```python
from build123d import *

# Parameters (mm, degrees)
SKETCH2_R               = 76.2
BOSS_EXTRUDE1_DEPTH     = 76.2
SKETCH21_R              = 2.6035
CUT_EXTRUDE4_DEPTH      = 9.525
SKETCH22_R              = 2.6035
CUT_EXTRUDE5_DEPTH      = 9.525
SKETCH27_W              = 38.1
SKETCH27_H              = 38.1
CUT_EXTRUDE7_DEPTH      = 50.8
SKETCH28_W              = 38.1
SKETCH28_H              = 38.1
CUT_EXTRUDE8_DEPTH      = 12.7
CUT_EXTRUDE8_DEPTH_BACK = 12.7
SKETCH29_W              = 50.8
SKETCH29_H              = 50.8
CUT_EXTRUDE9_DEPTH      = 63.5
SKETCH30_R              = 9.525
CUT_EXTRUDE10_DEPTH     = 19.05


with BuildPart() as part:
    # Sketch1 → Revolve1 (revolve)
    with BuildSketch(Plane.XY):
        with BuildLine():
            Line((78.359, 0), (0, 0))
            Line((0, 0), (0, 254))
            add(Edge.make_bspline(
                [(78.359, 0), (78.359, 0.547287489), (78.357845602, 1.649563618), (78.352650776, 3.586349875), (78.338796346, 5.988934596), (78.318010672, 8.352211569), (78.29028895, 10.745600888), (78.246958697, 13.731411826), (78.181061307, 17.311703382), (78.08386626, 21.490442467), (77.944822085, 26.264117007), (77.777683186, 31.037557631), (77.58229134, 35.809557456), (77.358460439, 40.580511863), (77.042853487, 46.542286246), (76.679080298, 52.501436144), (76.266448568, 58.457359127), (75.804102806, 64.409607399), (75.404015228, 69.168949637), (74.865626928, 75.114798701), (74.157385744, 82.243973993), (73.238266918, 90.551730955), (72.055740597, 100.030771811), (70.735528943, 109.491671534), (69.270929118, 118.931305028), (67.249996919, 130.699881306), (64.501732948, 144.763840427), (61.308555538, 158.735984092), (57.591049496, 172.577213574), (53.383025938, 186.275905479), (49.238746312, 198.044837449), (44.48323743, 209.587335711), (38.942884235, 220.71924179), (34.256173135, 228.693595393), (29.818710248, 235.095423042), (25.624249732, 240.182852143), (21.978892835, 243.926180276), (18.570150197, 246.859542723), (15.474349081, 249.076247661), (12.563405711, 250.785701438), (9.772327363, 252.083533871), (7.063069709, 253.028642362), (4.275373805, 253.686778481), (2.188006886, 253.939891173), (0.767171586, 253.999916555), (0, 254)],
                knots=[0.083290168, 0.083290168, 0.083290168, 0.083290168, 0.083290168, 0.091119674, 0.09894918, 0.106778686, 0.114608192, 0.122437698, 0.130267203, 0.145926215, 0.161585227, 0.177244239, 0.192903251, 0.208562263, 0.224221275, 0.239880287, 0.27119831, 0.286857322, 0.302516334, 0.318175346, 0.333834359, 0.365152383, 0.396470407, 0.42778843, 0.459106453, 0.490424474, 0.521742495, 0.584378539, 0.647014581, 0.678332609, 0.709650637, 0.772286631, 0.810589211, 0.841907031, 0.872607503, 0.893486158, 0.91262845, 0.928287274, 0.941044948, 0.952387223, 0.962498308, 0.97249612, 0.981348672, 0.989949856, 1, 1, 1, 1, 1], degree=4))
        make_face()
    revolve(axis=Axis((0, 254, 0), (0, -1, 0)))

    # Sketch2 → Boss-Extrude1 (add)
    with BuildSketch(Plane.XZ):
        Circle(SKETCH2_R)
    extrude(amount=BOSS_EXTRUDE1_DEPTH)

    # Sketch21 → Cut-Extrude4 (cut)
    with BuildSketch(Plane.XZ.offset(76.2)):
        with Locations((-37.81298, 0)):
            Circle(SKETCH21_R)
        with Locations((0, 37.81298)):
            Circle(SKETCH21_R)
        with Locations((37.81298, 0)):
            Circle(SKETCH21_R)
        with Locations((0, -37.81298)):
            Circle(SKETCH21_R)
    extrude(amount=-CUT_EXTRUDE4_DEPTH, mode=Mode.SUBTRACT)

    # Sketch22 → Cut-Extrude5 (cut)
    with BuildSketch(Plane.XZ.offset(76.2)):
        with Locations((-35.921024484, -35.921024484)):
            Circle(SKETCH22_R)
        with Locations((-35.921024484, 35.921024484)):
            Circle(SKETCH22_R)
        with Locations((35.921024484, 35.921024484)):
            Circle(SKETCH22_R)
        with Locations((35.921024484, -35.921024484)):
            Circle(SKETCH22_R)
    extrude(amount=-CUT_EXTRUDE5_DEPTH, mode=Mode.SUBTRACT)

    # Sketch27 → Cut-Extrude7 (cut)
    with BuildSketch(Plane(origin=(0, 44.016832576, -17.279280796), x_dir=(-1, 0, 0), z_dir=(0, -0.930845359, 0.365413352))):
        with Locations((-26.421293772, -9.04130389)):
            Rectangle(SKETCH27_W, SKETCH27_H)
        with Locations((37.219487863, -8.332945695)):
            Rectangle(SKETCH27_W, SKETCH27_H)
        with Locations((-23.648296478, -56.578488001)):
            Rectangle(SKETCH27_W, SKETCH27_H)
        with Locations((24.603212251, -57.8468214)):
            Rectangle(SKETCH27_W, SKETCH27_H)
    extrude(amount=-CUT_EXTRUDE7_DEPTH, mode=Mode.SUBTRACT)

    # Sketch28 → Cut-Extrude8 (cut, two sides)
    with BuildSketch(Plane(origin=(0, 20.37336046, -7.997781656), x_dir=(-1, 0, 0), z_dir=(0, -0.930845359, 0.365413352))) as cut_extrude8_sk:
        with Locations((-22.607200089, 28.533823854)):
            Rectangle(SKETCH28_W, SKETCH28_H)
        with Locations((33.495403265, 12.697844386)):
            Rectangle(SKETCH28_W, SKETCH28_H)
        with Locations((-27.648315988, -27.501194113)):
            Rectangle(SKETCH28_W, SKETCH28_H)
        with Locations((21.868067431, -36.368513827)):
            Rectangle(SKETCH28_W, SKETCH28_H)
    extrude(amount=CUT_EXTRUDE8_DEPTH, mode=Mode.SUBTRACT)
    extrude(cut_extrude8_sk.sketch, amount=-CUT_EXTRUDE8_DEPTH_BACK, mode=Mode.SUBTRACT)

    # Sketch29 → Cut-Extrude9 (cut)
    with BuildSketch(Plane(origin=(0, 109.036380897, -42.80340343), x_dir=(-1, 0, 0), z_dir=(0, -0.930845359, 0.365413352))):
        with Locations((-4.810844723, -59.078878237)):
            Rectangle(SKETCH29_W, SKETCH29_H)
    extrude(amount=-CUT_EXTRUDE9_DEPTH, mode=Mode.SUBTRACT)

    # Sketch30 → Cut-Extrude10 (cut)
    with BuildSketch(Plane.XZ.offset(76.2)):
        Circle(SKETCH30_R)
    extrude(amount=-CUT_EXTRUDE10_DEPTH, mode=Mode.SUBTRACT)


solid = part.part
```
CAD build for the part. Positions are in the model's coordinates, mm. Round coordinates to 2 decimals unless told otherwise and drop trailing zeros. Order: outer loops, then holes, each group sorted by start corner. A loop starts at its lowest first (then second) coordinate and runs counter-clockwise, first axis right, second up. Notation, with made-up numbers: (40.5, 55) - (83.5, 55) arc R30 ccw to (83.5, 83) - close; hole circle Ø4 at (70, 11.5). An arc over 180 degrees is marked (long way). Use CSV: the item, a comma, the result in double quotes. Start each with the question number.
1) Pin check, flat tips, straight feed: pin 1 Ø2 at (y, z) = (97.5, 52) entering from -X; pin 2 Ø10 at (x, y) = (-60.5, 17) entering from +Z; pin 3 Ø2.5 at (x, z) = (35.5, 36) entering from -Y (3 decimals). Stop position of each tip, or through.
2) Saw through at A-A (y = -32.5). List the corners of the cut face in (x, z).
3) Wall check: L1, parallel to Z at x = 0, y = -66.75 (3 decimals); L2, parallel to Z at x = -8, y = 95.5; L3, parallel to Z at x = -11, y = 162.5. Give the ranges that are in metal, low to high. Write a range as [from, to].
4) Saw through at B-B (x = -24). Count the separate pieces of the cut face and the enclosed holes in it, and give its area (3 significant figures).
5) Two-plate mould, pull along Z, no slides. Class faces 1 (the flat face through (16, -76.2, 1)), 2 (the cylindrical face through (-7.559, -66.808, -5.796)): pulls with the +Z half, pulls with the -Z half, needs draft (parallel to the pull), parting line crosses it, or undercut.
Values follow:
1,pin 1,"stops at x = -51.34"
1,pin 2,"stops at z = 55.07"
1,pin 3,"stops at y = -66.675"
2,outline,"circle Ø152.4 at (0, 0)"
3,L1,"z = [-76.2, -40.416], [-35.209, -9.525], [9.525, 35.209], [40.416, 76.2]"
3,L2,"z = [-72.17, 4.19], [45.12, 72.17]"
3,L3,"z = [-59.21, -27.61], [26.96, 59.21]"
4,separate pieces,"1"
4,enclosed holes,"4"
4,area,"33,500 mm2"
5,face 1,"needs draft"
5,face 2,"undercut"
